from build123d import *

# Parameters (mm, degrees)
F1_DEPTH = 30
F2_R     = 4.4
F3_R     = 4.4
F4_DEPTH = 25
F5_R     = 2
F6_R     = 2


# Not quite as in the source:
# - a feature names something its author has since deleted; it is built from what else it names


with BuildPart() as f1:
    # F0 (on Front) → F1 (new body)
    with BuildSketch(Plane.XZ):
        Polygon((90, -1), (90, 1), (70, 1), (70, 59), (-70, 59), (-70, 1), (-90, 1), (-90, -1), (-68, -1), (-68, 57), (68, 57), (68, -1), align=None)
    extrude(amount=F1_DEPTH)

    # F2 (on face) + F3 (on face) → F4 (cut)
    with BuildSketch(Plane.XY.offset(1)):
        with Locations((-80, -15)):
            Circle(F2_R)
        with Locations((80, -15)):
            Circle(F2_R)
    with BuildSketch(Plane.XY.offset(59)):
        with Locations((-25, -15)):
            Circle(F3_R)
        with Locations((25, -15)):
            Circle(F3_R)
    extrude(amount=-F4_DEPTH, mode=Mode.SUBTRACT)

    # F5
    f5_edges = [f1.edges().sort_by_distance(p)[0] for p in [
        (-70, -15, 59),
        (70, -15, 59),
    ]]
    fillet(f5_edges, radius=F5_R)

    # F6
    f6_edges = [f1.edges().sort_by_distance(p)[0] for p in [
        (68, -15, -1),
        (-68, -15, -1),
    ]]
    fillet(f6_edges, radius=F6_R)


solid = f1.part
Geometry check sheet. Reference: the model listing, model coordinates, mm. A direction names the side the tool comes from. Round coordinates to 2 decimals unless told otherwise and drop trailing zeros. Order: outer loops, then holes, each group sorted by start corner. A loop starts at its lowest first (then second) coordinate and runs counter-clockwise, first axis right, second up. Notation, with made-up numbers: M 66,72 L 124,72 A20 cw 124,77 Z; hole C 64,76 d11. An arc over 180 degrees is marked long. Answer in a Markdown table with one row per item.
(1) Sectioned sample at C-C, the plane x = 80. Record the cut outline in (y, z), and give its area (3 significant figures).
Responses:
| item | result |
|---|---|
| outline | M -30,-1 L -19.4,-1 L -19.4,1 L -30,1 Z; M -10.6,-1 L 0,-1 L 0,1 L -10.6,1 Z |
| area | 42.4 mm² |
(2) Sectioned sample at D-D, the plane y = -25.25. Record the cut outline in (x, z), and give its area (3 significant figures).
Responses:
| item | result |
|---|---|
| outline | M -90,-1 L -70,-1 A2 ccw -68,1 L -68,57 L 68,57 L 68,1 A2 ccw 70,-1 L 90,-1 L 90,1 L 70,1 L 70,57 A2 ccw 68,59 L -68,59 A2 ccw -70,57 L -70,1 L -90,1 Z |
| area | 589 mm² |
(3) Scan lines: probe 1 along Y at (x, z) = (25, 57.5); probe 2 along X at (y, z) = (-21, 32.5); probe 3 along Z at (x, y) = (-17, -10). Record each from-to range of solid material in increasing order. Write a range as from..to.
Responses:
| item | result |
|---|---|
| probe 1 | y = -30..-19.4, -10.6..0 |
| probe 2 | x = -70..-68, 68..70 |
| probe 3 | z = 57..59 |
(4) Sectioned sample at B-B, the plane y = -15. State how many separate pieces and enclosed holes the cut face has, and give its area (3 significant figures).
Responses:
| item | result |
|---|---|
| separate pieces | 5 |
| enclosed holes | 0 |
| area | 518 mm² |
(5) Tool access check on faces 4 (the face through (-75, -15, 1)), 5 (the face through (-22.635, -11.29, 58.014)), 6 (the face through (70, -15, 29)), 7 (the face through (68, -15, 29)). Record the directions out of +Z, -Z, +X, -X, +Y, -Y that give a thin tool (end or side, any length) a straight path to the whole face; none if there is none.
Responses:
| item | result |
|---|---|
| face 4 | +Z, -X, +Y, -Y |
| face 5 | +Z, -Z |
| face 6 | +Z, +X, +Y, -Y |
| face 7 | -Z, +Y, -Y |
(6) Sectioned sample at A-A, the plane z = 29.5. Record the cut outline in (x, y), and give its area (3 significant figures).
Responses:
| item | result |
|---|---|
| outline | M -70,-30 L -68,-30 L -68,0 L -70,0 Z; M 68,-30 L 70,-30 L 70,0 L 68,0 Z |
| area | 120 mm² |
(7) Go/stop test with flat-tipped pins: P1, Ø12, axis at y = -17, z = 39, coming from the +X side; P2, Ø14, axis at x = 80, y = -15, coming from the +Z side; P3, Ø2, axis at y = -26, z = 26, coming from the -X side. Record where each tip stops, or that it passes through.
Responses:
| item | result |
|---|---|
| P1 | stops at x = 70 |
| P2 | stops at z = 1 |
| P3 | stops at x = -70 |
(8) Draft check along Y on faces 1 (the face through (-84.396, -14.807, 0.014)), 2 (the face through (85, -15, 1)), 3 (the face through (0, 0, 58)). Enter one of: released by +Y, released by -Y, zero draft, split by the parting line, or undercut.
Responses:
| item | result |
|---|---|
| face 1 | undercut |
| face 2 | zero draft |
| face 3 | released by +Y |
